Autodesk Inventor part; units mm, degrees
ref_plane "YZ Plane" through (0, 0, 0) normal (1, 0, 0) x (0, 1, 0)
ref_plane "XZ Plane" through (0, 0, 0) normal (0, 1, 0) x (-1, 0, 0)
ref_plane "XY Plane" through (0, 0, 0) normal (0, 0, 1) x (1, 0, 0)
sketch "Sketch1" plane through (0, 0, 0) normal (0, 0, 1) x (1, 0, 0)
  line L0 (-270.2344, -114.33) -> (-270.2344, -13.08)
  circle A0 centre (-227.9995, -79.405) radius 7.5
  circle A1 centre (-134.4524, -69.88) radius 7.5
  circle A2 centre (-54.3408, -69.88) radius 15.875
  circle A3 centre (-54.3408, -46.8612) radius 2.3813
  circle A4 centre (-31.322, -69.88) radius 2.3813
  circle A5 centre (-77.3595, -69.88) radius 2.3813
  circle A6 centre (-54.3408, -92.8987) radius 2.3813
  line L1 (-270.2344, -13.08) -> (5.175, -13.08)
  line L2 (-270.2344, -114.33) -> (5.1968, -114.33)
  line L3 (280.6281, -114.33) -> (280.6281, -13.08)
  line L4 (280.6281, -13.08) -> (5.175, -13.08)
  line L5 (280.6281, -114.33) -> (5.1968, -114.33)
  line L6 (-285.2344, 1.92) -> (295.5844, 1.92)
  line L7 (295.5844, 1.92) -> (295.5844, -129.33)
  line L8 (295.5844, -129.33) -> (-285.2344, -129.33)
  line L9 (-285.2344, -129.33) -> (-285.2344, 1.92)
  line L10 (-59, 1.92) -> (-59, 25.92)
  line L11 (-285.2344, -38) -> (-309.2344, -38)
  line L12 (-43, -129.33) -> (-43, -153.33)
  line L13 (295.5844, -72.2612) -> (319.5844, -72.2612)
  line L14 (-309.2344, 25.92) -> (319.6281, 25.92)
  line L15 (319.6281, 25.92) -> (319.6281, -153.33)
  line L16 (319.6281, -153.33) -> (-309.2344, -153.33)
  line L17 (-309.2344, -153.33) -> (-309.2344, 25.92)
  line L18 (2, -13.08) -> (2, 1.92)
  line L19 (5.175, -13.08) -> (5.175, 1.92)
  line L20 (2, -129.33) -> (2, -114.33)
  line L21 (-285.2344, -56.825) -> (-270.2344, -56.825)
  line L22 (-285.2344, -60) -> (-270.2344, -60)
  line L23 (280.6281, -56.825) -> (295.5844, -56.825)
  line L24 (5.1968, -114.33) -> (5.175, -129.33)
  line L25 (280.6281, -60) -> (295.5844, -60)
  circle A7 centre (238.3931, -79.405) radius 7.5
  circle A8 centre (144.846, -69.88) radius 7.5
  circle A9 centre (64.7344, -69.88) radius 15.875
  circle A10 centre (64.7344, -46.8612) radius 2.3813
  circle A11 centre (41.7157, -69.88) radius 2.3813
  circle A12 centre (87.7532, -69.88) radius 2.3813
  circle A13 centre (64.7344, -92.8987) radius 2.3813
  circle A14 centre (64.7344, -69.88) radius 38.1
  circle A15 centre (-54.3408, -69.88) radius 38.1
  point P0 (0, 0)
  dimension "d4" = 15
  dimension "d7" = 15
  dimension "d9" = 31.75
  dimension "d11" = 4.7625
  dimension "d13" = 4.7625
  dimension "d15" = 23.0188
  dimension "d16" = 4.7625
  dimension "d18" = 4.7625
  dimension "d25" = 550.8625
  dimension "d30" = 24
  dimension "d31" = 24
  dimension "d32" = 24
  dimension "d33" = 24
  dimension "d34" = 3.175
  dimension "d36" = 3.175
  dimension "d50" = 23.0188
  dimension "d51" = 23.0188
  dimension "d52" = 23.0188
  dimension "d53" = 80.1116
  dimension "d54" = 93.5471
  dimension "d56" = 119.0752
  dimension "d57" = 80.1116
  dimension "d60" = 93.5471
  dimension "d61" = 76.2
  dimension "d62" = 76.2
extrude "Extrusion2" add sketch "Sketch1" along normal blind 9.525 contours L0 L1 L4 L3 L5 L2 | L22 L9 L21 L0 | L2 L24 L8 L20 | L9 L8 L12 L16 L17 L11 | L8 L7 L6 L10 L14 L15 L16 L12 | L18 L6 L19 L1 | L11 L17 L14 L10 L6 L9 | L3 L23 L7 L25 | A14 | A15
emboss "Emboss2" sketch "Sketch1" operation cut depth 3 direction (0, 0, 1) contours A14 | A15
properties part number "side-UPDATED"
Can you work these out from the model? Positions are in its coordinate system, mm. A direction names the side the tool comes from. Coordinates: 2 decimals unless noted, no trailing zeros. Write each loop counter-clockwise with the first axis right and the second up, starting at its lowest first coordinate (ties: lowest second). Pieces come first, ordered by that corner, then holes. Notation, with made-up numbers: (-25.75, -22.75) -> (24.25, -22.75) arc R16 cw to (24.25, -6.75) -> close; hole circle Ø1 at (41.5, -8). An arc over 180 degrees is marked (long way). Answer as CSV lines item,"result".
1) If I drill on line 1 (X direction, y = -124, z = 5); line 2 (Y direction, x = -202.5, z = 2.25); line 3 (X direction, y = -43.5, z = 4), over which ranges is the centre line in solid material (lowest first)? Write a range as from..to.
Check result:
line 1,"-309.23..-285.23, 2..5.18, 295.58..319.63"
line 2,"-153.33..-129.33, -114.33..-13.08, 1.92..25.92"
line 3,"-309.23..-285.23, -270.23..280.63, 295.58..319.63"
2) If we section it at A-A on y = -22: Please give me the cut outline in (x, z) (3 decimals).
Check result:
outline,"(-309.234, 0) -> (-285.234, 0) -> (-285.234, 9.525) -> (-309.234, 9.525) -> close; (-270.234, 0) -> (280.628, 0) -> (280.628, 9.525) -> (-270.234, 9.525) -> close; (295.584, 0) -> (319.628, 0) -> (319.628, 9.525) -> (295.584, 9.525) -> close"
3) If we section it at C-C on z = 7.75: Count the separate pieces of the cut face and the enclosed holes in it, then the cut area to 3 significant figures.
Check result:
separate pieces,"1"
enclosed holes,"18"
area,"90,000 mm²"
4) Will this pin go through, and if not, where does the flat tip stop? P1, Ø6, axis at x = -54.34, y = -46.86, coming from the -Z side.
Check result:
P1,"z = 3"
5) If we section it at B-B on x = 190.5: Please give me the cut outline in (y, z) (3 decimals).
Check result:
outline,"(-153.33, 0) -> (-129.33, 0) -> (-129.33, 9.525) -> (-153.33, 9.525) -> close; (-114.33, 0) -> (-13.08, 0) -> (-13.08, 9.525) -> (-114.33, 9.525) -> close; (1.92, 0) -> (25.92, 0) -> (25.92, 9.525) -> (1.92, 9.525) -> close"
6) If we mould it in two halves opening along Y, with no side actions, what happens to faces 1 (the cylindrical face through (79.4, -63.8, 6.2)), 2 (the flat face through (1, -62, 9.525)), 3 (the cylindrical face through (26.67, -71.56, 1.48))? For each: +Y half, -Y half, draft (parallel to the pull), parting line (faces both ways), or undercut.
Check result:
face 1,"undercut"
face 2,"draft"
face 3,"undercut"
7) On a 3-axis mill with a long thin cutter (end or side, diameter ignored), from which of +Z, -Z, +X, -X, +Y, -Y can I reach the whole of each face in a straight line? I mean faces 4 (the cylindrical face through (-127.299, -72.133, 4.696)), 5 (the flat face through (-55, -86, 3)). Say none if no direction works.
Check result:
face 4,"+Z, -Z"
face 5,"-Z"
